Could you check a few things on this model? Use its own coordinates, in mm. Round coordinates to 2 decimals unless told otherwise and drop trailing zeros. Loops run counter-clockwise (first coordinate to the right, second up) from the corner with the lowest first, then second, coordinate; pieces in that order, holes last. Notation, with made-up numbers: (75.25, 72.25) -> (89.25, 72.25) arc R33 cw to (89.25, 106.25) -> close; hole circle Ø11 at (36.25, 44). An arc over 180 degrees is marked (long way). Put each result on its own line as item: value. Start each with the question number.
1. Imagine slicing it at C-C, the plane x = 49. Please give me the cut outline in (y, z), and give its area (3 significant figures).
2. Imagine slicing it at A-A, the plane z = 25. Please give me the cut outline in (x, y).
3. Imagine slicing it at B-B, the plane x = -25. Please give me the cut outline in (y, z), and give its area (3 significant figures).
4. I'm going to push a flat-ended pin straight in: P1, Ø4, axis at x = 55, z = -25, coming from the +Y side. Where does the tip first touch, or does it pass through?
5. I need wall thicknesses on line 1 (Z direction, x = -55, y = 2.25); line 2 (X direction, y = 0.65, z = -25); line 3 (Z direction, x = 36.5, y = 2.85). Which ranges of each line are inside material? Lowest first, please. Write a range as [from, to].
6. Imagine slicing it at D-D, the plane y = 2.15. Count the separate pieces of the cut face and the enclosed holes in it, and give its area (3 significant figures).
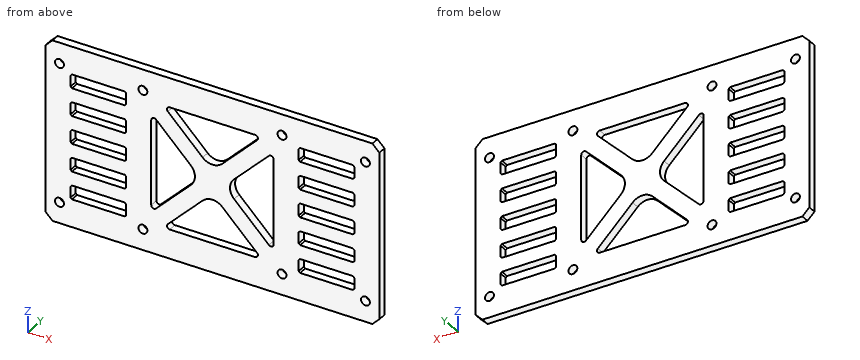
```python
from build123d import *

# Parameters (mm, degrees)
SKETCH_1_W          = 120
SKETCH_1_H          = 65
SKETCH_1_R          = 1.6
EXTRUDE_1_DEPTH     = 3
CUT_EXTRUDE_1_REACH = 5
SKETCH_2_R          = 1.6
CUT_EXTRUDE_2_REACH = 5
CUT_EXTRUDE_3_DEPTH = 3
CHAMFER_1_SIZE      = 2.5


with BuildPart() as part:
    # 草图1 → 凸台-拉伸1 (new body)
    with BuildSketch(Plane(origin=(0, 0, 0), x_dir=(1, 0, 0), z_dir=(0, 1, 0))):
        Rectangle(SKETCH_1_W, SKETCH_1_H)
        with Locations((-25, 25)):
            Circle(SKETCH_1_R, mode=Mode.SUBTRACT)
        with Locations((25, 25)):
            Circle(SKETCH_1_R, mode=Mode.SUBTRACT)
        with Locations((25, -25)):
            Circle(SKETCH_1_R, mode=Mode.SUBTRACT)
        with Locations((-25, -25)):
            Circle(SKETCH_1_R, mode=Mode.SUBTRACT)
    extrude(amount=EXTRUDE_1_DEPTH)

    # 草图2 → 切除-拉伸1 (cut, up to next)
    with BuildSketch(Plane(origin=(0, 3, 0), x_dir=(1, 0, 0), z_dir=(0, 1, 0)), mode=Mode.PRIVATE) as cut_extrude_1_sk1:
        with Locations((55, 25)):
            Circle(SKETCH_2_R)
    cut_extrude_1_tool1 = extrude(cut_extrude_1_sk1.sketch, amount=-CUT_EXTRUDE_1_REACH, mode=Mode.PRIVATE) & part.part
    add(cut_extrude_1_tool1.solids().sort_by_distance((55, 3, -25))[0], mode=Mode.SUBTRACT)
    # 草图2 → 切除-拉伸1 (cut, up to next)
    with BuildSketch(Plane(origin=(0, 3, 0), x_dir=(1, 0, 0), z_dir=(0, 1, 0)), mode=Mode.PRIVATE) as cut_extrude_1_sk2:
        with Locations((55, -25)):
            Circle(SKETCH_2_R)
    cut_extrude_1_tool2 = extrude(cut_extrude_1_sk2.sketch, amount=-CUT_EXTRUDE_1_REACH, mode=Mode.PRIVATE) & part.part
    add(cut_extrude_1_tool2.solids().sort_by_distance((55, 3, 25))[0], mode=Mode.SUBTRACT)
    # 草图2 → 切除-拉伸1 (cut, up to next)
    with BuildSketch(Plane(origin=(0, 3, 0), x_dir=(1, 0, 0), z_dir=(0, 1, 0)), mode=Mode.PRIVATE) as cut_extrude_1_sk3:
        with Locations((-55, -25)):
            Circle(SKETCH_2_R)
    cut_extrude_1_tool3 = extrude(cut_extrude_1_sk3.sketch, amount=-CUT_EXTRUDE_1_REACH, mode=Mode.PRIVATE) & part.part
    add(cut_extrude_1_tool3.solids().sort_by_distance((-55, 3, 25))[0], mode=Mode.SUBTRACT)
    # 草图2 → 切除-拉伸1 (cut, up to next)
    with BuildSketch(Plane(origin=(0, 3, 0), x_dir=(1, 0, 0), z_dir=(0, 1, 0)), mode=Mode.PRIVATE) as cut_extrude_1_sk4:
        with Locations((-55, 25)):
            Circle(SKETCH_2_R)
    cut_extrude_1_tool4 = extrude(cut_extrude_1_sk4.sketch, amount=-CUT_EXTRUDE_1_REACH, mode=Mode.PRIVATE) & part.part
    add(cut_extrude_1_tool4.solids().sort_by_distance((-55, 3, -25))[0], mode=Mode.SUBTRACT)

    # 草图3 → 切除-拉伸2 (cut, up to next)
    with BuildSketch(Plane(origin=(0, 3, 0), x_dir=(1, 0, 0), z_dir=(0, 1, 0)), mode=Mode.PRIVATE) as cut_extrude_2_sk1:
        with BuildLine():
            Line((-22, 15.343145751), (-22, -15.343145751))
            ThreePointArc((-22, -15.343145751), (-21.382683432, -16.267025283), (-20.292893219, -16.050252532))
            Line((-20.292893219, -16.050252532), (-7.778174593, -3.535533906))
            ThreePointArc((-7.778174593, -3.535533906), (-6.313708499, 0), (-7.778174593, 3.535533906))
            Line((-7.778174593, 3.535533906), (-20.292893219, 16.050252532))
            ThreePointArc((-20.292893219, 16.050252532), (-21.382683432, 16.267025283), (-22, 15.343145751))
        make_face()
    cut_extrude_2_tool1 = extrude(cut_extrude_2_sk1.sketch, amount=-CUT_EXTRUDE_2_REACH, mode=Mode.PRIVATE) & part.part
    add(cut_extrude_2_tool1.solids().sort_by_distance((-16.215858, 3, 0))[0], mode=Mode.SUBTRACT)
    # 草图3 → 切除-拉伸2 (cut, up to next)
    with BuildSketch(Plane(origin=(0, 3, 0), x_dir=(1, 0, 0), z_dir=(0, 1, 0)), mode=Mode.PRIVATE) as cut_extrude_2_sk2:
        with BuildLine():
            Line((15.343145751, 22), (-15.343145751, 22))
            ThreePointArc((-15.343145751, 22), (-16.267025283, 21.382683432), (-16.050252532, 20.292893219))
            Line((-16.050252532, 20.292893219), (-3.535533906, 7.778174593))
            ThreePointArc((-3.535533906, 7.778174593), (0, 6.313708499), (3.535533906, 7.778174593))
            Line((3.535533906, 7.778174593), (16.050252532, 20.292893219))
            ThreePointArc((16.050252532, 20.292893219), (16.267025283, 21.382683432), (15.343145751, 22))
        make_face()
    cut_extrude_2_tool2 = extrude(cut_extrude_2_sk2.sketch, amount=-CUT_EXTRUDE_2_REACH, mode=Mode.PRIVATE) & part.part
    add(cut_extrude_2_tool2.solids().sort_by_distance((0, 3, -16.215858))[0], mode=Mode.SUBTRACT)
    # 草图3 → 切除-拉伸2 (cut, up to next)
    with BuildSketch(Plane(origin=(0, 3, 0), x_dir=(1, 0, 0), z_dir=(0, 1, 0)), mode=Mode.PRIVATE) as cut_extrude_2_sk3:
        with BuildLine():
            Line((22, -15.343145751), (22, 15.343145751))
            ThreePointArc((22, 15.343145751), (21.382683432, 16.267025283), (20.292893219, 16.050252532))
            Line((20.292893219, 16.050252532), (7.778174593, 3.535533906))
            ThreePointArc((7.778174593, 3.535533906), (6.313708499, 0), (7.778174593, -3.535533906))
            Line((7.778174593, -3.535533906), (20.292893219, -16.050252532))
            ThreePointArc((20.292893219, -16.050252532), (21.382683432, -16.267025283), (22, -15.343145751))
        make_face()
    cut_extrude_2_tool3 = extrude(cut_extrude_2_sk3.sketch, amount=-CUT_EXTRUDE_2_REACH, mode=Mode.PRIVATE) & part.part
    add(cut_extrude_2_tool3.solids().sort_by_distance((16.215858, 3, 0))[0], mode=Mode.SUBTRACT)
    # 草图3 → 切除-拉伸2 (cut, up to next)
    with BuildSketch(Plane(origin=(0, 3, 0), x_dir=(1, 0, 0), z_dir=(0, 1, 0)), mode=Mode.PRIVATE) as cut_extrude_2_sk4:
        with BuildLine():
            Line((-15.343145751, -22), (15.343145751, -22))
            ThreePointArc((15.343145751, -22), (16.267025283, -21.382683432), (16.050252532, -20.292893219))
            Line((16.050252532, -20.292893219), (3.535533906, -7.778174593))
            ThreePointArc((3.535533906, -7.778174593), (0, -6.313708499), (-3.535533906, -7.778174593))
            Line((-3.535533906, -7.778174593), (-16.050252532, -20.292893219))
            ThreePointArc((-16.050252532, -20.292893219), (-16.267025283, -21.382683432), (-15.343145751, -22))
        make_face()
    cut_extrude_2_tool4 = extrude(cut_extrude_2_sk4.sketch, amount=-CUT_EXTRUDE_2_REACH, mode=Mode.PRIVATE) & part.part
    add(cut_extrude_2_tool4.solids().sort_by_distance((0, 3, 16.215858))[0], mode=Mode.SUBTRACT)

    # 草图4 → 切除-拉伸3 (cut)
    with BuildSketch(Plane.XZ):
        Polygon((50.5, -2.5), (51, -2), (51, 2), (50.5, 2.5), (31.5, 2.5), (31, 2), (31, -2), (31.5, -2.5), align=None)
        Polygon((50.5, 7.5), (31.5, 7.5), (31, 8), (31, 12), (31.5, 12.5), (50.5, 12.5), (51, 12), (51, 8), align=None)
        Polygon((50.5, 17.5), (31.5, 17.5), (31, 18), (31, 22), (31.5, 22.5), (50.5, 22.5), (51, 22), (51, 18), align=None)
        Polygon((31.5, -17.5), (31, -18), (31, -22), (31.5, -22.5), (50.5, -22.5), (51, -22), (51, -18), (50.5, -17.5), align=None)
        Polygon((31.5, -7.5), (31, -8), (31, -12), (31.5, -12.5), (50.5, -12.5), (51, -12), (51, -8), (50.5, -7.5), align=None)
        Polygon((-50.5, -7.5), (-31.5, -7.5), (-31, -8), (-31, -12), (-31.5, -12.5), (-50.5, -12.5), (-51, -12), (-51, -8), align=None)
        Polygon((-50.5, -17.5), (-31.5, -17.5), (-31, -18), (-31, -22), (-31.5, -22.5), (-50.5, -22.5), (-51, -22), (-51, -18), align=None)
        Polygon((-31.5, 17.5), (-31, 18), (-31, 22), (-31.5, 22.5), (-50.5, 22.5), (-51, 22), (-51, 18), (-50.5, 17.5), align=None)
        Polygon((-31.5, 7.5), (-31, 8), (-31, 12), (-31.5, 12.5), (-50.5, 12.5), (-51, 12), (-51, 8), (-50.5, 7.5), align=None)
        Polygon((-31.5, 2.5), (-31, 2), (-31, -2), (-31.5, -2.5), (-50.5, -2.5), (-51, -2), (-51, 2), (-50.5, 2.5), align=None)
    extrude(amount=-CUT_EXTRUDE_3_DEPTH, mode=Mode.SUBTRACT)

    # 倒角1
    chamfer_1_edges = [part.edges().sort_by_distance(p)[0] for p in [
        (60, 1.5, 32.5),
        (-60, 1.5, 32.5),
        (-60, 1.5, -32.5),
        (60, 1.5, -32.5),
    ]]
    chamfer(chamfer_1_edges, length=CHAMFER_1_SIZE)


solid = part.part
```
Entries:
1. outline: (0, -32.5) -> (3, -32.5) -> (3, -22.5) -> (0, -22.5) -> close; (0, -17.5) -> (3, -17.5) -> (3, -12.5) -> (0, -12.5) -> close; (0, -7.5) -> (3, -7.5) -> (3, -2.5) -> (0, -2.5) -> close; (0, 2.5) -> (3, 2.5) -> (3, 7.5) -> (0, 7.5) -> close; (0, 12.5) -> (3, 12.5) -> (3, 17.5) -> (0, 17.5) -> close; (0, 22.5) -> (3, 22.5) -> (3, 32.5) -> (0, 32.5) -> close
1. area: 120 mm^2
2. outline: (-60, 0) -> (-56.6, 0) -> (-56.6, 3) -> (-60, 3) -> close; (-53.4, 0) -> (-26.6, 0) -> (-26.6, 3) -> (-53.4, 3) -> close; (-23.4, 0) -> (23.4, 0) -> (23.4, 3) -> (-23.4, 3) -> close; (26.6, 0) -> (53.4, 0) -> (53.4, 3) -> (26.6, 3) -> close; (56.6, 0) -> (60, 0) -> (60, 3) -> (56.6, 3) -> close
3. outline: (0, -32.5) -> (3, -32.5) -> (3, -26.6) -> (0, -26.6) -> close; (0, -23.4) -> (3, -23.4) -> (3, 23.4) -> (0, 23.4) -> close; (0, 26.6) -> (3, 26.6) -> (3, 32.5) -> (0, 32.5) -> close
3. area: 176 mm^2
4. P1: y = 3
5. line 1: [-32.5, -26.6], [-23.4, 23.4], [26.6, 32.5]
5. line 2: [-60, -56.6], [-53.4, -26.6], [-23.4, 23.4], [26.6, 53.4], [56.6, 60]
5. line 3: [-32.5, -22.5], [-17.5, -12.5], [-7.5, -2.5], [2.5, 7.5], [12.5, 17.5], [22.5, 32.5]
6. separate pieces: 1
6. enclosed holes: 22
6. area: 5,500 mm^2
